```python
from build123d import *

# Parameters (mm, degrees)
SKETCH1_W           = 6.35
SKETCH1_H           = 50.8
SKETCH1_W_2         = 63.5
SKETCH1_H_2         = 6.35
BOSS_EXTRUDE1_DEPTH = 508
SKETCH2_W           = 31.75
SKETCH2_H           = 6.35
REVOLVE2_ANGLE      = 180
SKETCH3_R           = 7.929881475
BOSS_EXTRUDE2_DEPTH = 44.45
SKETCH4_R           = 4.30972172
CUT_EXTRUDE1_DEPTH  = 44.45


with BuildPart() as part:
    # Sketch1 → Boss-Extrude1 (new body)
    with BuildSketch(Plane(origin=(0, 0, 0), x_dir=(1, 0, 0), z_dir=(0, 1, 0))):
        with Locations((3.175, 25.4)):
            Rectangle(SKETCH1_W, SKETCH1_H)
        with Locations((38.1, 47.625)):
            Rectangle(SKETCH1_W_2, SKETCH1_H_2)
        Polygon((69.85, 50.8), (69.85, 44.45), (69.85, 0), (76.2, 0), (76.2, 50.8), align=None)
    extrude(amount=BOSS_EXTRUDE1_DEPTH)

    # Sketch2 → Revolve2 (revolve)
    with BuildSketch(Plane.XZ):
        with Locations((22.225, -47.625)):
            Rectangle(SKETCH2_W, SKETCH2_H)
        Polygon((6.35, 0), (0, 0), (0, -50.8), (6.35, -50.8), (6.35, -44.45), align=None)
    revolve(axis=Axis((38.1, 0, -50.8), (0, 0, 1)), revolution_arc=REVOLVE2_ANGLE)

    # Sketch3 → Boss-Extrude2 (add)
    with BuildSketch(Plane.XY.offset(-44.45)):
        with Locations(Location((38.1, 0, 0), (0, 0, 180))):
            Circle(SKETCH3_R)
    extrude(amount=BOSS_EXTRUDE2_DEPTH)

    # Sketch4 → Cut-Extrude1 (cut)
    with BuildSketch(Plane.XY):
        with Locations((38.1, 0)):
            Circle(SKETCH4_R)
    extrude(amount=-CUT_EXTRUDE1_DEPTH, mode=Mode.SUBTRACT)


solid = part.part
```
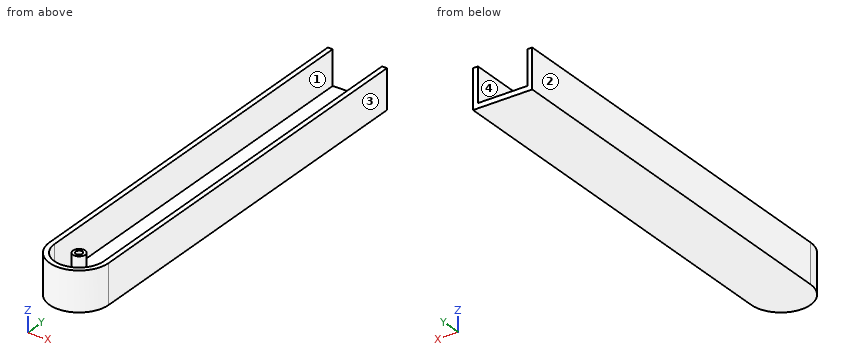
Part model, mm, in its own coordinate system. Face numbers are marked on the shaded views. Round coordinates to 2 decimals unless told otherwise and drop trailing zeros. Order: outer loops, then holes, each group sorted by start corner. A loop starts at its lowest first (then second) coordinate and runs counter-clockwise, first axis right, second up. Notation, with made-up numbers: M 76.25,72.25 L 108.25,72.25 A16 ccw 108.25,98.25 Z; hole C 10,-7.5 d3. An arc over 180 degrees is marked long. Put each result on its own line as item: value. Start each with the question number.
1. Drill centre lines: probe 1 along X at (y, z) = (52, -10); probe 2 along Y at (x, z) = (34.5, -25.5). Where is each one in solid material? Low to high. Write a range as [from, to].
2. Two-plate mould, pull along X, no slides. Class the marked faces 1, 2, 3 and 4: +X half, -X half, draft (parallel to the pull), parting line (faces both ways), or undercut.
3. Slice it at A-A on z = -40. List the corners of the cut face in (x, y), then the cut area to 3 significant figures.
4. Drop flat-ended pins along their axis: pin 1 (1.5 mm diameter, centred on x = 16, z = -22.5, fed in from -Y); pin 2 (4 mm diameter, centred on x = 54.5, z = -24, fed in from -Y); pin 3 (1 mm diameter, centred on x = 28.5, z = -23.5, fed in from -Y). Give the stop position or say it passes through.
5. Slice it at B-B on y = 327. List the corners of the cut face in (x, z), then the cut area to 3 significant figures.
6. Slice it at C-C on x = 61.5. List the corners of the cut face in (y, z), then the cut area to 3 significant figures.
Findings:
1. probe 1: [0, 6.35], [69.85, 76.2]
1. probe 2: [-37.93, -31.55], [-7.07, -2.37], [2.37, 7.07]
2. face 1: undercut
2. face 2: -X half
2. face 3: +X half
2. face 4: undercut
3. outline: M 0,0 A38.1 ccw 76.2,0 L 76.2,508 L 69.85,508 L 69.85,0 A31.75 cw 6.35,0 L 6.35,508 L 0,508 Z; C 38.1,0 d15.86; hole C 38.1,0 d8.62
3. area: 7,290 mm2
4. pin 1: y = -31.56
4. pin 2: y = -35.27
4. pin 3: y = -37
5. outline: M 0,-50.8 L 76.2,-50.8 L 76.2,0 L 69.85,0 L 69.85,-44.45 L 6.35,-44.45 L 6.35,0 L 0,0 Z
5. area: 1,050 mm2
6. outline: M -30.07,-50.8 L 508,-50.8 L 508,-44.45 L -21.46,-44.45 L -21.46,0 L -30.07,0 Z
6. area: 3,800 mm2
